from build123d import *

# Parameters (mm, degrees)
SKETCH1_R           = 29
SKETCH1_R_2         = 26.9
EXTRUDE1_DEPTH      = 40
EXTRUDE2_DEPTH      = 7.3
EXTRUDE2_DEPTH_BACK = 8
SKETCH2_R           = 27.05
SKETCH2_R_2         = 24.7
THREAD1_PITCH       = 2
THREAD1_FROM        = 2
CHAMFER1_SIZE       = 0.5
CHAMFER2_SIZE       = 2.5
CHAMFER4_SIZE       = 0.25


with BuildPart() as part:
    # Sketch1 → Extrude1 (new body)
    with BuildSketch(Plane.XY):
        Circle(SKETCH1_R)
        Circle(SKETCH1_R_2, mode=Mode.SUBTRACT)
    extrude(amount=EXTRUDE1_DEPTH)

    # Sketch2 → Extrude2 (add, two sides: drawn at the far end of the back side and taken through both)
    with BuildSketch(Plane.XY.offset(40).offset(-EXTRUDE2_DEPTH_BACK)):
        Circle(SKETCH2_R)
        Circle(SKETCH2_R_2, mode=Mode.SUBTRACT)
    extrude(amount=EXTRUDE2_DEPTH + EXTRUDE2_DEPTH_BACK)

    # Thread1: arcs per turn and ends read off the stored shape
    # Thread1: the profile of Sketch4 profile screwed along a right-hand helix through 4.65 turns, 10 arcs to a turn; built about Z, then put on its axis
    thread1_z = Axis((0, 0, 0), (0, 0, 1))
    thread1_corners = [(27.0497, 0, -0.000173205), (27.591265875, 0, 0.312499999), (27.591265875, 0, 0.437499999), (27.0497, 0, 0.750173202)]
    with BuildLine(mode=Mode.PRIVATE) as thread1_profile:
        Line(thread1_corners[0], thread1_corners[1])
        Line(thread1_corners[1], thread1_corners[2])
        Line(thread1_corners[2], thread1_corners[3])
        Line(thread1_corners[3], thread1_corners[0])
    thread1_cap = Face(thread1_profile.wire())
    thread1_turn_angles = [0, 18, 36, 54, 72, 90, 108, 126, 144, 162, 180, 198, 216, 234, 252, 270, 288, 306, 324, 342, 360]
    thread1_turn_weights = [1, 0.9510565162951535, 1, 0.9510565162951535, 1, 0.9510565162951535, 1, 0.9510565162951535, 1, 0.9510565162951535, 1, 0.9510565162951535, 1, 0.9510565162951535, 1, 0.9510565162951535, 1, 0.9510565162951535, 1, 0.9510565162951535, 1]
    thread1_turn_rails = [Edge.make_bspline([Vector(p[0], p[1], 0).rotate(thread1_z, thread1_turn_angles[k]) / thread1_turn_weights[k] + Vector(0, 0, p[2] + THREAD1_PITCH * thread1_turn_angles[k] / 360) for k in range(21)], [0, 0, 0, 1, 1, 2, 2, 3, 3, 4, 4, 5, 5, 6, 6, 7, 7, 8, 8, 9, 9, 10, 10, 10], 2, thread1_turn_weights) for p in thread1_corners]
    thread1_turn_sides = [Face.make_surface_from_curves(thread1_turn_rails[p[0]], thread1_turn_rails[p[1]]) for p in [(0, 1), (1, 2), (2, 3), (3, 0)]]
    thread1_last_angles = [1440, 1458, 1476, 1494, 1512, 1530, 1548, 1566, 1584, 1602, 1620, 1638, 1656, 1665, 1674]
    thread1_last_weights = [1, 0.9510565162951535, 1, 0.9510565162951535, 1, 0.9510565162951535, 1, 0.9510565162951535, 1, 0.9510565162951535, 1, 0.9510565162951535, 1, 0.9876883405951371, 1]
    thread1_last_rails = [Edge.make_bspline([Vector(p[0], p[1], 0).rotate(thread1_z, thread1_last_angles[k]) / thread1_last_weights[k] + Vector(0, 0, p[2] + THREAD1_PITCH * thread1_last_angles[k] / 360) for k in range(15)], [0, 0, 0, 1, 1, 2, 2, 3, 3, 4, 4, 5, 5, 6, 6, 7, 7, 7], 2, thread1_last_weights) for p in thread1_corners]
    thread1_last_sides = [Face.make_surface_from_curves(thread1_last_rails[p[0]], thread1_last_rails[p[1]]) for p in [(0, 1), (1, 2), (2, 3), (3, 0)]]
    thread1 = Plane(origin=(0, 0, 49.3), x_dir=(-1, 0, 0), z_dir=(0, 0, -1)) * split(Solid(Shell([*[p.moved(Location((0, 0, THREAD1_PITCH * i))) for i in range(4) for p in thread1_turn_sides], *thread1_last_sides, thread1_cap, thread1_cap.rotate(thread1_z, 1674).moved(Location((0, 0, THREAD1_PITCH * 1674 / 360)))])), bisect_by=Plane.XY.offset(THREAD1_FROM), keep=Keep.TOP, mode=Mode.PRIVATE)
    add(thread1)

    # Chamfer1
    chamfer1_edges = [part.edges().sort_by_distance(p)[0] for p in [
        (-24.7, 0, 47.3),
        (-29, 0, 40),
    ]]
    chamfer(chamfer1_edges, length=CHAMFER1_SIZE)

    # Chamfer2
    # the kernel refuses this chamfer: 2.5 mm, written as the material it takes off along each edge
    with BuildSketch(Plane(origin=(0, 0, 32), x_dir=(1, 0, 0), z_dir=(0, -1, 0))) as chamfer2_piece_1_section:
        Polygon((24.7 + CHAMFER2_SIZE, 0), (24.7, CHAMFER2_SIZE), (24.7, 0), align=None)
    chamfer2_piece_1 = revolve(axis=Axis((0, 0, 32), (0, 0, 1)), mode=Mode.PRIVATE)
    chamfer2_piece_1 = chamfer2_piece_1 & Plane(origin=(0, 0, 32), x_dir=(1, 0, 0), z_dir=(0, 0, -1)) * Cylinder(26.9, 109, mode=Mode.PRIVATE)
    add(chamfer2_piece_1, mode=Mode.SUBTRACT)

    # Sketch7 → Cut-Revolve1 (revolve, cut)
    with BuildSketch(Plane(origin=(0, 0, 0), x_dir=(1, 0, 0), z_dir=(0, 1, 0))):
        Polygon((-28.009015865, -45.840984135), (-26.55, -47.3), (-27.05, -47.3), (-28.680601357, -47.3), (-28.680601357, -45.840984135), align=None)
    revolve(axis=Axis((0, 0, 0), (0, 0, 1)), mode=Mode.SUBTRACT)

    # Chamfer4
    chamfer4_edges = [part.edges().sort_by_distance(p)[0] for p in [
        (-26.9, 0, 0),
    ]]
    chamfer(chamfer4_edges, length=CHAMFER4_SIZE)


solid = part.part
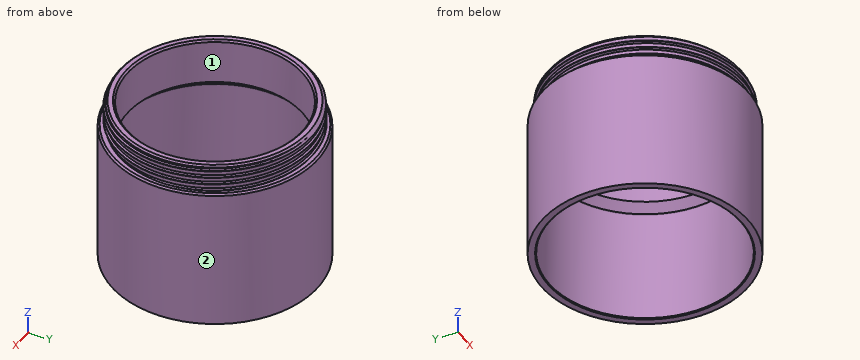
Read the model definition and answer for the solid it produces. Units are mm, in the model's axes. Face numbers are marked on the shaded views. Give positions to 0.01 mm unless a question says otherwise; leave off trailing zeros. Write each loop counter-clockwise with the first axis right and the second up, starting at its lowest first coordinate (ties: lowest second). Pieces come first, ordered by that corner, then holes. Notation, with made-up numbers: (35.25, -40) - (86.25, -40) arc R33 ccw to (86.25, -3) - close; hole circle Ø4 at (-3.75, 31). An arc over 180 degrees is marked (long way). Answer in a Markdown table with one row per item. Add a question column.
Item 1: Section A-A, the plane z = 35.5 is taken. Write down the section's boundary in (x, y), and give its area (3 significant figures).
Item 2: Find the intervals of material crossed by L1, parallel to Y at x = 0, z = 13; L2, parallel to X at y = -17, z = 10.5; L3, parallel to X at y = 13, z = 14, in increasing order.
Item 3: Flat-ended cylindrical pins translate along their axes: P1, Ø3, axis at y = 17, z = 17.5, coming from the +X side; P2, Ø6, axis at y = -13, z = 23, coming from the +X side; P3, Ø3, axis at x = 5.5, z = 19, coming from the -Y side. Find the tip coordinate at first contact, or state that the pin passes through.
Item 4: Section B-B, the plane z = 13.5 is taken. Write down the section's boundary in (x, y), and give its area (3 significant figures).
Item 5: Determine the mould class of the marked faces 1 and 2 for opening direction X: pulls with the +X half, pulls with the -X half, needs draft (parallel to the pull), parting line crosses it, or undercut.
Recorded:
| question | item | result |
|---|---|---|
| 1 | outline | circle Ø58 at (0, 0); hole circle Ø49.4 at (0, 0) |
| 1 | area | 725 mm2 |
| 2 | L1 | y = -29 to -26.9, 26.9 to 29 |
| 2 | L2 | x = -23.49 to -20.85, 20.85 to 23.49 |
| 2 | L3 | x = -25.92 to -23.55, 23.55 to 25.92 |
| 3 | P1 | stops at x = 24.51 |
| 3 | P2 | stops at x = 27.22 |
| 3 | P3 | stops at y = -28.72 |
| 4 | outline | circle Ø58 at (0, 0); hole circle Ø53.8 at (0, 0) |
| 4 | area | 369 mm2 |
| 5 | face 1 | undercut |
| 5 | face 2 | parting line crosses it |
